Read the model definition and answer for the solid it produces. Units are mm, in the model's axes. A direction names the side the tool comes from. Round coordinates to 2 decimals unless told otherwise and drop trailing zeros. Loops run counter-clockwise (first coordinate to the right, second up) from the corner with the lowest first, then second, coordinate; pieces in that order, holes last. Notation, with made-up numbers: M 17.5,11.5 L 46.5,11.5 A21 cw 46.5,44.5 Z; hole C 48,67.5 d2. An arc over 180 degrees is marked long. Answer as CSV lines item,"result".
```python
from build123d import *

# Parameters (mm, degrees)
BOSS_EXTRUDE1_DEPTH             = 3
CUT_EXTRUDE1_REACH              = 35.675
SKETCH2_R                       = 1.3750000000000009
BOSS_EXTRUDE2_REACH             = 35.675
BOSS_EXTRUDE2_DIRECTION_2_REACH = 35.675
FILLET3_R                       = 1
FILLET3_OF_MIRROR2_R            = 1
FILLET6_R                       = 5
FILLET7_R                       = 1


with BuildPart() as part:
    # Sketch1 → Boss-Extrude1 (new body)
    with BuildSketch(Plane(origin=(0, 0, 0), x_dir=(1, 0, 0), z_dir=(0, 1, 0))):
        Polygon((30, -14.999999999999993), (-29.999999999999996, -15.000000000000002), (-29.999999999999996, 14.999999999999998), (30.000000000000004, 15.000000000000005), align=None)
    extrude(amount=BOSS_EXTRUDE1_DEPTH)

    # Sketch2 → Cut-Extrude1 (cut, up to next)
    with BuildSketch(Plane(origin=(0, 3, 0), x_dir=(1, 0, 0), z_dir=(0, 1, 0)), mode=Mode.PRIVATE) as cut_extrude1_sk1:
        with Locations(Location((-18.5, 0, 0), (0, 0, 270))):
            Circle(SKETCH2_R)
    cut_extrude1_tool1 = extrude(cut_extrude1_sk1.sketch, amount=-CUT_EXTRUDE1_REACH, mode=Mode.PRIVATE) & part.part
    cut_extrude1 = cut_extrude1_tool1.solids().sort_by_distance((-18.5, 3, 0))[0]
    add(cut_extrude1, mode=Mode.SUBTRACT)

    # Mirror1: Cut-Extrude1 across plane
    add(cut_extrude1.mirror(Plane(origin=(0, 0, 0), x_dir=(0, 0, 1), z_dir=(1, 0, 0))), mode=Mode.SUBTRACT)

    # Boss-Extrude2: up to this face of the body (flat: up to its plane)
    boss_extrude2_end = Plane(part.part.faces().sort_by_distance((0, 1.5, 15))[0])
    # Sketch3 → Boss-Extrude2 (add, up to the picked face)
    with BuildSketch(Plane.XY, mode=Mode.PRIVATE) as boss_extrude2_sk1:
        with BuildLine():
            Line((24.23371870266459, 15.000000000000002), (21.01832839349107, 3))
            Line((21.01832839349107, 3), (30, 3))
            Line((30, 3), (29.999999999999996, 11.500000000107407))
            ThreePointArc((29.999999999999996, 11.500000000107407), (32.223130931464034, 11.891997965331278), (34.17811946267373, 13.020711120091907))
            Line((34.17811946267373, 13.020711120091907), (33.213938048141515, 14.169777784768357))
            ThreePointArc((33.213938048141515, 14.169777784768357), (25.019026509541703, 17.564221286256522), (32.50000000000003, 22.3301270189222))
            Line((32.50000000000003, 22.3301270189222), (33.250000000000036, 23.62916512459886))
            ThreePointArc((33.250000000000036, 23.62916512459886), (25.505721350569345, 22.695898148519827), (24.23371870266459, 15.000000000000002))
        make_face()
    boss_extrude2_tool1 = split(extrude(boss_extrude2_sk1.sketch, amount=BOSS_EXTRUDE2_REACH, mode=Mode.PRIVATE), bisect_by=boss_extrude2_end, keep=Keep.BOTH, mode=Mode.PRIVATE)
    boss_extrude2 = boss_extrude2_tool1.solids().sort_by(Axis((26.59731, 11.034621, 0), (0, 0, 1)))[0]
    add(boss_extrude2)

    # Boss-Extrude2 direction 2: up to this face of the body (flat: up to its plane)
    boss_extrude2_direction_2_end = Plane(part.part.faces().sort_by_distance((0, 1.5, -15))[0])
    # Sketch3 → Boss-Extrude2 direction 2 (add, up to the picked face)
    with BuildSketch(Plane.XY, mode=Mode.PRIVATE) as boss_extrude2_direction_2_sk1:
        with BuildLine():
            Line((24.23371870266459, 15.000000000000002), (21.01832839349107, 3))
            Line((21.01832839349107, 3), (30, 3))
            Line((30, 3), (29.999999999999996, 11.500000000107407))
            ThreePointArc((29.999999999999996, 11.500000000107407), (32.223130931464034, 11.891997965331278), (34.17811946267373, 13.020711120091907))
            Line((34.17811946267373, 13.020711120091907), (33.213938048141515, 14.169777784768357))
            ThreePointArc((33.213938048141515, 14.169777784768357), (25.019026509541703, 17.564221286256522), (32.50000000000003, 22.3301270189222))
            Line((32.50000000000003, 22.3301270189222), (33.250000000000036, 23.62916512459886))
            ThreePointArc((33.250000000000036, 23.62916512459886), (25.505721350569345, 22.695898148519827), (24.23371870266459, 15.000000000000002))
        make_face()
    boss_extrude2_direction_2_tool1 = split(extrude(boss_extrude2_direction_2_sk1.sketch, amount=-BOSS_EXTRUDE2_DIRECTION_2_REACH, mode=Mode.PRIVATE), bisect_by=boss_extrude2_direction_2_end, keep=Keep.BOTH, mode=Mode.PRIVATE)
    boss_extrude2_direction_2 = boss_extrude2_direction_2_tool1.solids().sort_by(Axis((26.59731, 11.034621, 0), (0, 0, -1)))[0]
    add(boss_extrude2_direction_2)

    # Fillet3
    # the kernel refuses this fillet: 1 mm, written as the material it adds along each edge
    with BuildSketch(Plane(origin=(29.999999999999996, 11.500000000107406, -15.000000000000002), x_dir=(0.9977653155349889, 0.06681597949116533, 0), z_dir=(0, 0, 1))) as fillet3_piece_1:
        with BuildLine():
            CenterArc((0.9354237099720605, -0.99776531555048), FILLET3_R, 93.83112782826316, 82.33774433018942)
            Line((-0.06234160556292847, -0.9309493360593146), (0, 0))
            ThreePointArc((0, 0), (0.4343038653561172, -0.01452544892746713), (0.8686077307122309, -1e-17))
        make_face()
    extrude(amount=30)
    # the kernel refuses this fillet: 1 mm, written as the material it takes off along each edge
    with BuildSketch(Plane(origin=(33.250000000000036, 23.62916512459886, 17.96693441323381), x_dir=(-0.9080543065649367, 0.4188524517403138, 0), z_dir=(0, 0, -1))) as fillet3_2_piece_1:
        with BuildLine():
            CenterArc((1.0954834756555598, -0.995824323371254), FILLET3_R, 84.76215915180506, 100.47568169639004)
            Line((0.09965915228430783, -1.0871146130092202), (0, 0))
            ThreePointArc((0, 0), (0.5933868826467665, 0.02714189808684594), (1.1867737652935233, 0))
        make_face()
    extrude(amount=35.93386882646762, mode=Mode.SUBTRACT)
    with BuildSketch(Plane(origin=(32.50000000000003, 22.3301270189222, -17.290199457863853), x_dir=(0.5000000000000039, 0.8660254037844365, 0), z_dir=(0, 0, 1))) as fillet3_2_piece_2:
        with BuildLine():
            CenterArc((0.9160797831455422, 0.9999999999999977), FILLET3_R, 189.59406822434758, 80.40593177565233)
            ThreePointArc((-0.06993351404503671, 0.8333333333765751), (-0.01751405270363253, 0.41813130141934185), (0, 0))
            Line((0, 0), (0.9160797831455412, -3e-17))
        make_face()
    extrude(amount=34.5803989157277, mode=Mode.SUBTRACT)
    with BuildSketch(Plane(origin=(34.17811946267373, 13.02071112009191, -17.96693441327771), x_dir=(-0.6427876096881444, 0.7660444431176312, 0), z_dir=(0, 0, 1))) as fillet3_2_piece_3:
        with BuildLine():
            CenterArc((1.0916730868583728, 1.0000000000000009), FILLET3_R, 169.52431830288586, 100.47568169711377)
            ThreePointArc((0.1083409208250382, 1.1818181818306124), (0.02714189812493758, 0.5933868826533465), (0, 0))
            Line((0, 0), (1.0916730868583666, -2e-17))
        make_face()
    extrude(amount=35.93386882655541, mode=Mode.SUBTRACT)
    with BuildSketch(Plane(origin=(33.213938048141515, 14.169777784768355, -17.29019945772614), x_dir=(-0.8171150585222966, -0.5764746144767381, 0), z_dir=(0, 0, 1))) as fillet3_2_piece_4:
        with BuildLine():
            CenterArc((0.9198888630675175, 0.9964971894548403), FILLET3_R, 184.7970341139915, 80.40593177249599)
            Line((-0.0766083263866242, 0.9128709291653951), (0, 0))
            ThreePointArc((0, 0), (0.4181313013932034, 0.01751405272528074), (0.8362626027864033, 2e-17))
        make_face()
    extrude(amount=34.58039891545228, mode=Mode.SUBTRACT)

    # Mirror2: Boss-Extrude2, Boss-Extrude2 direction 2 across plane
    add(boss_extrude2.mirror(Plane(origin=(0, 0, 0), x_dir=(0, 0, 1), z_dir=(1, 0, 0))))
    add(boss_extrude2_direction_2.mirror(Plane(origin=(0, 0, 0), x_dir=(0, 0, 1), z_dir=(1, 0, 0))))

    # Fillet3 of Mirror2
    # the kernel refuses this fillet: 1 mm, written as the material it adds along each edge
    with BuildSketch(Plane(origin=(-29.999999999999996, 11.500000000107406, 14.999999999999998), x_dir=(-0.9977653155349889, 0.06681597949116533, 0), z_dir=(0, 0, -1))) as fillet3_of_mirror2_piece_1:
        with BuildLine():
            CenterArc((0.9354237099720605, -0.99776531555048), FILLET3_OF_MIRROR2_R, 93.83112782826316, 82.33774433018942)
            Line((-0.06234160556292847, -0.9309493360593146), (0, 0))
            ThreePointArc((0, 0), (0.4343038653561172, -0.01452544892746713), (0.8686077307122309, -1e-17))
        make_face()
    extrude(amount=30)
    # the kernel refuses this fillet: 1 mm, written as the material it takes off along each edge
    with BuildSketch(Plane(origin=(-33.250000000000036, 23.629165124598856, 17.966934413233812), x_dir=(0.5000000000000044, -0.866025403784436, 0), z_dir=(0, 0, -1))) as fillet3_of_mirror2_2_piece_1:
        with BuildLine():
            CenterArc((1.0916730868040134, -1.0000000000000007), FILLET3_OF_MIRROR2_R, 90.00000000000007, 100.47568169639015)
            ThreePointArc((0.10834092076838271, -1.181818181818188), (0.02714189808684512, -0.5933868826467682), (0, 0))
            Line((0, 0), (1.091673086804012, -2e-17))
        make_face()
    extrude(amount=35.93386882646763, mode=Mode.SUBTRACT)
    with BuildSketch(Plane(origin=(-32.50000000000003, 22.3301270189222, 17.29019945786385), x_dir=(0.9048050109861938, 0.42582612894733674, 0), z_dir=(0, 0, -1))) as fillet3_of_mirror2_2_piece_2:
        with BuildLine():
            CenterArc((0.9198888631228366, -0.996497189454418), FILLET3_OF_MIRROR2_R, 94.79703411380164, 80.40593177565235)
            Line((-0.07660832633633094, -0.9128709292248977), (0, 0))
            ThreePointArc((0, 0), (0.41813130141834665, -0.01751405272739198), (0.8362626028366937, -2e-17))
        make_face()
    extrude(amount=34.5803989157277, mode=Mode.SUBTRACT)
    with BuildSketch(Plane(origin=(-34.17811946267373, 13.020711120091908, 17.966934413277702), x_dir=(0.8215259563306123, -0.5701711173630887, 0), z_dir=(0, 0, -1))) as fillet3_of_mirror2_2_piece_3:
        with BuildLine():
            CenterArc((1.0954834757069158, -0.995824323374353), FILLET3_OF_MIRROR2_R, 84.76215915375006, 100.47568169711377)
            Line((0.09965915233991275, -1.0871146130587033), (0, 0))
            ThreePointArc((0, 0), (0.59338688265553, 0.02714189807715625), (1.1867737653110744, 8e-17))
        make_face()
    extrude(amount=35.9338688265554, mode=Mode.SUBTRACT)
    with BuildSketch(Plane(origin=(-33.213938048141515, 14.169777784768355, 17.290199457726136), x_dir=(-0.6427876096881426, -0.7660444431176326, 0), z_dir=(0, 0, -1))) as fillet3_of_mirror2_2_piece_4:
        with BuildLine():
            CenterArc((0.916079783090449, -1.0000000000000009), FILLET3_OF_MIRROR2_R, 89.99999999999977, 80.40593177249599)
            ThreePointArc((-0.06993351409094786, -0.8333333333222552), (-0.01751405272878019, -0.4181313013930569), (0, 0))
            Line((0, 0), (0.916079783090453, 2e-17))
        make_face()
    extrude(amount=34.58039891545228, mode=Mode.SUBTRACT)

    # Fillet6
    fillet6_edges = [part.edges().sort_by_distance(p)[0] for p in [
        (30, 0, -5.33e-15),
        (-29.999999999999996, 0, 1.78e-15),
    ]]
    fillet(fillet6_edges, radius=FILLET6_R)

    # Fillet7
    fillet7_edges = [part.edges().sort_by_distance(p)[0] for p in [
        (21.01832839349107, 3, -1.78e-15),
        (24.23371870266459, 15.000000000000004, -1.78e-15),
        (-24.23371870266459, 15.000000000000004, -1.78e-15),
        (-21.01832839349107, 3, -1.78e-15),
    ]]
    fillet(fillet7_edges, radius=FILLET7_R)


solid = part.part
```
1) Find section A-A, the plane x = 18.5. Give the vertices of the cut face in (y, z) (3 decimals), then the cut area to 4 significant figures.
Evaluation:
outline,"M 0,-15 L 3,-15 L 3,-1.375 L 0,-1.375 Z; M 0,1.375 L 3,1.375 L 3,15 L 0,15 Z"
area,"81.75 mm^2"
2) Each of these flat-tipped pins is pushed along its axis until it touches: P1, Ø3, axis at y = 6.5, z = -1, coming from the -X side; P2, Ø9, axis at x = 30, y = 18, coming from the +Z side; P3, Ø3.5, axis at x = -18.5, z = 0, coming from the +Y side; P4, Ø3, axis at y = 5, z = 3, coming from the +X side. Where does it stop, or does it pass through?
Evaluation:
P1,"stops at x = -30"
P2,"passes through"
P3,"stops at y = 3"
P4,"stops at x = 30"
3) Find section C-C, the plane z = -11.5. Give the vertices of the cut face in (x, y), then the cut area to 3 significant figures.
Evaluation:
outline,"M -33.61,13.64 A1 ccw -33.2,12.34 A6.5 ccw -30.87,11.56 A1 cw -30,10.57 L -30,5 A5 ccw -25,0 L 25,0 A5 ccw 30,5 L 30,10.57 A1 cw 30.87,11.56 A6.5 ccw 33.2,12.34 A1 ccw 33.61,13.64 A1 ccw 32.53,13.69 A5 cw long 31.74,22.69 A1 ccw 32.8,22.92 A1 ccw 32.17,24.13 A6.5 ccw 24.08,15.31 A1 cw 24.14,14.64 L 21.22,3.74 A1 cw 20.25,3 L -20.25,3 A1 cw -21.22,3.74 L -24.14,14.64 A1 cw -24.08,15.31 A6.5 ccw -32.17,24.13 A1 ccw -32.8,22.92 A1 ccw -31.74,22.69 A5 cw long -32.53,13.69 A1 ccw Z"
area,"392 mm^2"
4) Determine the mould class of faces 4 (the cylindrical face through (17.137, 1.521, -0.179)), 5 (the cylindrical face through (32.056, 11.834, 0.21)), 6 (the cylindrical face through (-32.73, 23.64, 0.21)), 7 (the flat face through (-1, 2, 15)) for opening direction X: released by +X, released by -X, zero draft, split by the parting line, or undercut.
Evaluation:
face 4,"undercut"
face 5,"released by +X"
face 6,"released by -X"
face 7,"zero draft"
5) A tool of negligible diameter and unlimited length cuts with its end or side. For faces 1 (the flat face through (-30, 8, 0)), 2 (the flat face through (30, 8, 0)), 3 (the flat face through (-22.7, 9.27, 0.21)), from which of +Z, -Z, +X, -X, +Y, -Y can it reach the whole face along a straight path? Write none if from no direction.
Evaluation:
face 1,"+Z, -Z, -X, -Y"
face 2,"+Z, -Z, +X, -Y"
face 3,"+Z, -Z"
6) Find section D-D, the plane z = 0. Count the separate pieces of the cut face and the enclosed holes in it, then the cut area to 3 significant figures.
Evaluation:
separate pieces,"3"
enclosed holes,"0"
area,"375 mm^2"
7) Straight lines are drawn through the part: line 1 (X direction, y = 2.15, z = 0) (3 decimals); line 2 (X direction, y = 2, z = 0) (3 decimals); line 3 (X direction, y = 18, z = 0.25). For each, find the intervals that lie inside material, in ascending order.
Evaluation:
line 1,"x = -29.108 to -19.875, -17.125 to 17.125, 19.875 to 29.108"
line 2,"x = -29 to -19.875, -17.125 to 17.125, 19.875 to 29"
line 3,"x = -25 to -23.5, 23.5 to 25"
8) Find section B-B, the plane y = 6.25. Give the vertices of the cut face in (x, z).
Evaluation:
outline,"M -30,-15 L -21.89,-15 L -21.89,15 L -30,15 Z; M 21.89,-15 L 30,-15 L 30,15 L 21.89,15 Z"
